from build123d import *

# Parameters (mm, degrees)
F0_W     = 85
F0_H     = 23
F0_H_2   = 40
F1_DEPTH = 3
F2_W     = 3
F2_H     = 23
F3_DEPTH = 24
F4_W     = 3
F4_H     = 23
F5_DEPTH = 25
F6_R     = 4
F7_DEPTH = 200


with BuildPart() as f1:
    # F0 (on Top) → F1 (new body)
    with BuildSketch(Plane.XY):
        with Locations((42.5, 11.5)):
            Rectangle(F0_W, F0_H)
        with Locations((42.5, -20)):
            Rectangle(F0_W, F0_H_2)
    extrude(amount=F1_DEPTH)

    # F2 (on face) → F3 (join)
    with BuildSketch(Plane.XY.offset(3)):
        with Locations((1.5, 11.5)):
            Rectangle(F2_W, F2_H)
        with Locations((83.5, 11.5)):
            Rectangle(F2_W, F2_H)
    extrude(amount=F3_DEPTH)

    # F4 (on face) → F5 (join)
    with BuildSketch(Plane.XY.offset(27)):
        with Locations((1.5, 11.5)):
            Rectangle(F4_W, F4_H)
    extrude(amount=F5_DEPTH)

    # F6 (on face) → F7 (cut)
    with BuildSketch(Plane.YZ.offset(85)):
        with Locations((11.5, 13.5)):
            Circle(F6_R)
    extrude(amount=-F7_DEPTH, mode=Mode.SUBTRACT)


solid = f1.part
Geometry: final body of the model. Coordinates: model frame, mm. A direction names the side the tool comes from. Coordinates: 2 decimals unless noted, no trailing zeros. Loops run counter-clockwise (first coordinate to the right, second up) from the corner with the lowest first, then second, coordinate; pieces in that order, holes last. Notation, with made-up numbers: M -15.5,0.25 L 4.5,0.25 A24 ccw 4.5,15.25 Z; hole C 54,62 d8. An arc over 180 degrees is marked long. One line per item, written item: value. Start each with the question number.
1) Reachability of faces 4 (the flat face through (3, 11, 27)), 5 (the flat face through (1, 0, 27)), 6 (the flat face through (83, 12, 27)), 7 (the flat face through (0, 5, 20)) from +Z, -Z, +X, -X, +Y, -Y: full face, straight path, thin tool, end or side. Return the list, or none.
2) Draft query along X for faces 1 (the flat face through (83, 0, 15)), 2 (the flat face through (82, 9, 17)), 3 (the flat face through (85, 5, 10)). Return one class per face: released by +X, released by -X, zero draft, split by the parting line, or undercut.
3) Cut plane B-B (z = 18.5). Return loops of the section in (x, y).
4) Pin query (flat end, axial travel): P1, Ø3.5, axis at x = 83.5, z = 18.5, coming from the -Y side; P2, Ø1.5, axis at x = 84, y = 16, coming from the +Z side; P3, Ø7, axis at y = 13.5, z = 38.5, coming from the +X side; P4, Ø6.5, axis at y = 11.5, z = 13.5, coming from the +X side. Return the tip coordinate at first contact, or that it passes through.
5) Material intervals for L1, parallel to X at y = 1, z = 18.5; L2, parallel to Z at x = 1, y = 11.5; L3, parallel to Z at x = 84.25, y = 11.5, sorted ascending. Write a range as from..to.
6) Cut plane D-D (z = 35.5). Return loops of the section in (x, y).
7) Cut plane A-A (y = 11.5). Return loops of the section in (x, z), then the cut area to 3 significant figures.
8) Cut plane C-C (x = 42.5). Return loops of the section in (y, z).
Evaluation:
1. face 4: +Z, +Y, -Y
1. face 5: +Z, +X, -X, -Y
1. face 6: +Z, +X, +Y, -Y
1. face 7: +Z, -Z, -X, +Y, -Y
2. face 1: zero draft
2. face 2: undercut
2. face 3: released by +X
3. outline: M 0,0 L 3,0 L 3,23 L 0,23 Z; M 82,0 L 85,0 L 85,23 L 82,23 Z
4. P1: y = 0
4. P2: z = 27
4. P3: x = 3
4. P4: through
5. L1: 0..3, 82..85
5. L2: 0..9.5, 17.5..52
5. L3: 0..9.5, 17.5..27
6. outline: M 0,0 L 3,0 L 3,23 L 0,23 Z
7. outline: M 0,0 L 85,0 L 85,9.5 L 82,9.5 L 82,3 L 3,3 L 3,9.5 L 0,9.5 Z; M 0,17.5 L 3,17.5 L 3,52 L 0,52 Z; M 82,17.5 L 85,17.5 L 85,27 L 82,27 Z
7. area: 426 mm^2
8. outline: M -40,0 L 23,0 L 23,3 L -40,3 Z
